Design review of the part built by this model. Coordinates are the model's own, in mm. A direction names the side the tool comes from. Give positions to 0.01 mm unless a question says otherwise; leave off trailing zeros. Order: outer loops, then holes, each group sorted by start corner. A loop starts at its lowest first (then second) coordinate and runs counter-clockwise, first axis right, second up. Notation, with made-up numbers: M 62,-29 L 80,-29 A26 cw 80,-12 Z; hole C 23.5,36 d3. An arc over 180 degrees is marked long. Answer as a JSON object with one key per item and string values.
Autodesk Fusion 360 part; units mm, degrees
sketch "Sketch1" plane through (0, 0, 0) normal (0, 0, 1) x (1, 0, 0)
  circle A0 centre (0, 0) radius 25
  dimension "d1" = 50
extrude "Extrude1" add sketch "Sketch1" along normal blind 2.5
sketch "Sketch2" plane through (0, 0, 2.5) normal (0, 0, 1) x (-1, 0, 0)
  circle A0 centre (0, 0) radius 25
  circle A1 centre (0, 0) radius 4
  line L0 (-6, 0) -> (-3, -5.1962) construction
  line L1 (-3, -5.1962) -> (3, -5.1962) construction
  line L2 (3, -5.1962) -> (6, 0) construction
  line L3 (6, 0) -> (3, 5.1962) construction
  line L4 (3, 5.1962) -> (-3, 5.1962) construction
  line L5 (-3, 5.1962) -> (-6, 0) construction
  circle A2 centre (0, 0) radius 21.75
  line L6 (-6, 0) -> (-21.75, 0)
  line L7 (6, 0) -> (21.75, 0)
  line L8 (-3, -5.1962) -> (-10.875, -18.8361)
  line L9 (3, -5.1962) -> (10.875, -18.8361)
  line L10 (-10.875, -18.8361) -> (-21.75, 0) construction
  line L11 (10.875, -18.8361) -> (21.75, 0) construction
  line L12 (-3, 5.1962) -> (-10.875, 18.8361)
  line L13 (3, 5.1962) -> (10.875, 18.8361)
  line L14 (10.875, 18.8361) -> (-10.875, 18.8361) construction
  line L15 (-21.75, 0) -> (-10.875, 18.8361) construction
  line L16 (-10.875, -18.8361) -> (10.875, -18.8361) construction
  circle A3 centre (0, 0) radius 6
  circle A4 centre (0, 0) radius 23
  dimension "d4" = 8
  dimension "d5" = 6
  dimension "d6" = 43.5
  dimension "d7" = 46
extrude "Extrude3" add sketch "Sketch2" along normal blind 1.5 contours A0 | A1 | A2 L7 L13 A3 | A2 L8 L9 A3 | A2 L6 L12 A3
(1) Draft analysis for pull direction X (two halves, no side actions). For faces 3 (the flat face through (-12, -7, 4)), 4 (the cylindrical face through (18.915, -10.737, 3.24)), state which applies: +X half, -X half, draft (parallel to the pull), parting line (faces both ways), or undercut.
Checked values:
{"face 3": "draft", "face 4": "undercut"}
(2) Tool access review of faces 1 (the flat face through (0, 15, 4)), 2 (the flat face through (-14, 0, 3)): name each direction out of +Z, -Z, +X, -X, +Y, -Y from which nothing blocks a thin tool from reaching the whole face with its end or side.
Checked values:
{"face 1": "+Z, +X, -X, +Y, -Y", "face 2": "+Z"}
(3) We need section A-A (y = -10). Write out the cut boundary in (x, z), plus the area to 3 significant figures.
Checked values:
{"outline": "M -22.91,0 L 22.91,0 L 22.91,4 L 20.71,4 L 20.71,2.5 L 19.31,2.5 L 19.31,4 L 5.77,4 L 5.77,2.5 L -5.77,2.5 L -5.77,4 L -19.31,4 L -19.31,2.5 L -20.71,2.5 L -20.71,4 L -22.91,4 Z", "area": "162 mm^2"}
(4) Insertion check: pin 1 (1.5 mm diameter, centred on x = -6.5, y = 6, fed in from -Z); pin 2 (1.6 mm diameter, centred on x = -10, z = 3.5, fed in from +Y); pin 3 (1 mm diameter, centred on y = -17, z = 1, fed in from -X); pin 4 (2 mm diameter, centred on y = 3.5, z = 2.5, fed in from -X). Each pin has a flat end and moves straight along its axis. Give the tip position at first contact, or say it passes through.
Checked values:
{"pin 1": "stops at z = 0", "pin 2": "stops at y = 23.25", "pin 3": "stops at x = -18.78", "pin 4": "stops at x = -24.87"}
(5) We need section B-B (z = 0.65). Write out the cut boundary in (x, y).
Checked values:
{"outline": "C 0,0 d50"}
(6) To check wall thickness, follow L1, parallel to Y at x = 0, z = 3.15; L2, parallel to X at y = 5.5, z = 3.3; L3, parallel to X at y = -10, z = 2.8. State the ranges of each line that lie inside material, in increasing order. Write a range as from..to.
Checked values:
{"L1": "y = -25..-23, -4..4, 6..21.75, 23..25", "L2": "x = -24.39..-22.33, -3.18..-2.4, 2.4..3.18, 22.33..24.39", "L3": "x = -22.91..-20.71, -19.31..-5.77, 5.77..19.31, 20.71..22.91"}
